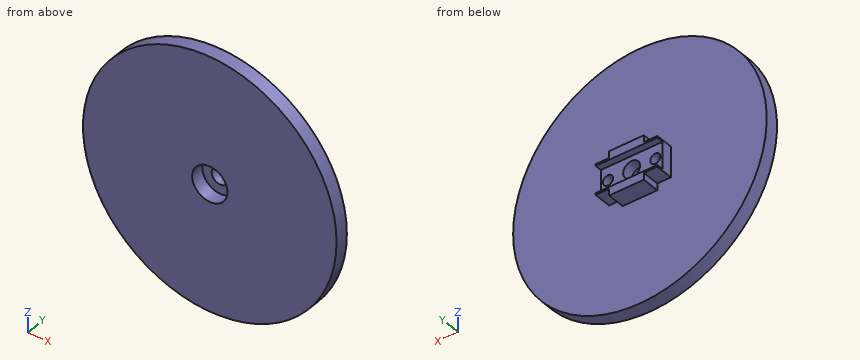
```python
from build123d import *

# Parameters (mm, degrees)
SKETCH1_R           = 37.5
BOSS_EXTRUDE1_DEPTH = 4
SKETCH2_R           = 5.22
CUT_EXTRUDE1_DEPTH  = 13.05
SKETCH3_W           = 18.27
SKETCH3_H           = 13.05
BOSS_EXTRUDE2_DEPTH = 5.22
SKETCH4_W           = 4
SKETCH4_H           = 2
CUT_EXTRUDE2_DEPTH  = 5.22
SKETCH5_W           = 53.664550202
SKETCH5_H           = 8
CUT_EXTRUDE3_DEPTH  = 2
SKETCH6_R           = 1.5
CUT_EXTRUDE4_DEPTH  = 4
SKETCH7_R           = 2.5
CUT_EXTRUDE5_DEPTH  = 8.22


with BuildPart() as part:
    # Sketch1 → Boss-Extrude1 (new body)
    with BuildSketch(Plane(origin=(0, 0, 0), x_dir=(1, 0, 0), z_dir=(0, 1, 0))):
        Circle(SKETCH1_R)
    extrude(amount=BOSS_EXTRUDE1_DEPTH)

    # Sketch2 → Cut-Extrude1 (cut)
    with BuildSketch(Plane(origin=(0, 4, 0), x_dir=(1, 0, 0), z_dir=(0, 1, 0))):
        Circle(SKETCH2_R)
    extrude(amount=-CUT_EXTRUDE1_DEPTH, mode=Mode.SUBTRACT)

    # Sketch3 → Boss-Extrude2 (add)
    with BuildSketch(Plane(origin=(0, 4, 0), x_dir=(1, 0, 0), z_dir=(0, 1, 0))):
        Rectangle(SKETCH3_W, SKETCH3_H)
    extrude(amount=BOSS_EXTRUDE2_DEPTH)

    # Sketch4 → Cut-Extrude2 (cut)
    with BuildSketch(Plane(origin=(0, 9.22, 0), x_dir=(1, 0, 0), z_dir=(0, 1, 0))):
        with Locations((-7.135, -5.525)):
            Rectangle(SKETCH4_W, SKETCH4_H)
        with Locations((-7.135, 5.525)):
            Rectangle(SKETCH4_W, SKETCH4_H)
        with Locations((7.135, 5.525)):
            Rectangle(SKETCH4_W, SKETCH4_H)
        with Locations((7.135, -5.525)):
            Rectangle(SKETCH4_W, SKETCH4_H)
    extrude(amount=-CUT_EXTRUDE2_DEPTH, mode=Mode.SUBTRACT)

    # Sketch5 → Cut-Extrude3 (cut)
    with BuildSketch(Plane(origin=(0, 9.22, 0), x_dir=(1, 0, 0), z_dir=(0, 1, 0))):
        Rectangle(SKETCH5_W, SKETCH5_H)
    extrude(amount=-CUT_EXTRUDE3_DEPTH, mode=Mode.SUBTRACT)

    # Sketch6 → Cut-Extrude4 (cut)
    with BuildSketch(Plane(origin=(0, 7.22, 0), x_dir=(1, 0, 0), z_dir=(0, 1, 0))):
        with Locations((-7, 0)):
            Circle(SKETCH6_R)
        with Locations((7, 0)):
            Circle(SKETCH6_R)
    extrude(amount=-CUT_EXTRUDE4_DEPTH, mode=Mode.SUBTRACT)

    # Sketch7 → Cut-Extrude5 (cut, through all)
    with BuildSketch(Plane(origin=(0, 7.22, 0), x_dir=(1, 0, 0), z_dir=(0, 1, 0))):
        Circle(SKETCH7_R)
    extrude(amount=-CUT_EXTRUDE5_DEPTH, mode=Mode.SUBTRACT)


solid = part.part
```
Part model, mm, in its own coordinate system. Give positions to 0.01 mm unless a question says otherwise; leave off trailing zeros. Order: outer loops, then holes, each group sorted by start corner. A loop starts at its lowest first (then second) coordinate and runs counter-clockwise, first axis right, second up. Notation, with made-up numbers: M 61.25,13 L 91.25,13 A29 ccw 91.25,35 Z; hole C 69,-14.75 d2. An arc over 180 degrees is marked long. Use a Markdown table: item, result. Add a question column.
(1) Probe line 1 along X through (y, z) = (5, 0) (3 decimals); line 2 along Z through (x, y) = (7, 4.95) (3 decimals); line 3 along Z through (x, y) = (0, 2.1). List the from-to ranges inside material, lowest first. Write a range as [from, to].
(2) Saw through at B-B, the plane y = 6. Give the cut face in (x, z) (3 decimals).
(3) Saw through at D-D, the plane z = -25.5. Give the cut face in (x, y), and give its area (3 significant figures).
(4) Drop flat-ended pins along their axis: P1, Ø4.5, axis at x = 7, y = 6.5, coming from the +Z side (3 decimals); P2, Ø0.6, axis at x = -2, y = 8.5, coming from the -Z side (3 decimals); P3, Ø22.5, axis at x = 8, z = 15.5, coming from the +Y side; P4, Ø4, axis at x = 24, z = 11, coming from the +Y side. Give the stop position or say it passes through.
(5) Saw through at C-C, the plane y = 2. Give the cut face in (x, z).
(6) Saw through at A-A, the plane x = 0. Give the cut face in (y, z) (3 decimals), and give its area (3 significant figures).
Answer key:
| question | item | result |
|---|---|---|
| 1 | line 1 | [-9.135, -8.5], [-5.5, -2.5], [2.5, 5.5], [8.5, 9.135] |
| 1 | line 2 | [-4.525, -1.5], [1.5, 4.525] |
| 1 | line 3 | [-37.5, -5.22], [5.22, 37.5] |
| 2 | outline | M -9.135,-4.525 L -5.135,-4.525 L -5.135,-6.525 L 5.135,-6.525 L 5.135,-4.525 L 9.135,-4.525 L 9.135,4.525 L 5.135,4.525 L 5.135,6.525 L -5.135,6.525 L -5.135,4.525 L -9.135,4.525 Z; hole C -7,0 d3; hole C 0,0 d5; hole C 7,0 d3 |
| 3 | outline | M -27.5,0 L 27.5,0 L 27.5,4 L -27.5,4 Z |
| 3 | area | 220 mm^2 |
| 4 | P1 | z = 6.525 |
| 4 | P2 | z = -6.525 |
| 4 | P3 | y = 9.22 |
| 4 | P4 | y = 4 |
| 5 | outline | C 0,0 d75; hole C 0,0 d10.44 |
| 6 | outline | M 0,-37.5 L 4,-37.5 L 4,-6.525 L 9.22,-6.525 L 9.22,-4 L 7.22,-4 L 7.22,-2.5 L 4,-2.5 L 4,-5.22 L 0,-5.22 Z; M 0,5.22 L 4,5.22 L 4,2.5 L 7.22,2.5 L 7.22,4 L 9.22,4 L 9.22,6.525 L 4,6.525 L 4,37.5 L 0,37.5 Z |
| 6 | area | 294 mm^2 |
